Input: part model. Units: mm. Frame: model coordinates. A direction names the side the tool comes from. Give positions to 0.01 mm unless a question says otherwise; leave off trailing zeros. Order: outer loops, then holes, each group sorted by start corner. A loop starts at its lowest first (then second) coordinate and runs counter-clockwise, first axis right, second up. Notation, with made-up numbers: (-24, 9) - (25, 9) arc R19 cw to (25, 20) - close; hole circle Ø2 at (44, 14.25). An arc over 180 degrees is marked (long way). Answer in a Markdown table with one row per item. Add a question column.
1. Access query for faces 1 (the face through (-6.952, 0.493, -0.434)), 2 (the face through (1, 1, -1)). Directions: +Z, -Z, +X, -X, +Y, -Y. A direction counts if a zero-diameter tool reaches every point of the face in a straight line with its end or side. Return the directions, or none.
2. Ray query, line 1 (Y direction, x = -15.5, z = -58); line 2 (X direction, y = 65, z = 0); line 3 (Z direction, x = 53, y = 79). Return the intervals inside material, ascending. Write a range as [from, to].
3. Section query C-C on y = 13. Return loops of the section in (x, z), and give its area (3 significant figures).
4. Section query A-A on z = 0. Return loops of the section in (x, y), and give its area (3 significant figures).
5. Contact query for flat-ended pins moving along their axis: pin 1 (12 mm diameter, centred on y = 36.5, z = 1, fed in from +X); pin 2 (1.5 mm diameter, centred on x = -15.5, z = 31.5, fed in from +Y); pin 3 (3 mm diameter, centred on x = 34, y = 19, fed in from -Z). Output: stop coordinate, or through.
6. Section query B-B on x = 0. Return loops of the section in (y, z).
7. Mould query, pull axis X, two halves, no side actions, for faces 3 (the face through (-48, 100, 53.4)), 4 (the face through (-1.2, 0.5, -6.6)), 5 (the face through (21.477, 49.807, 68.198)), 6 (the face through (21.78, 49.3, 69.15)). Classes: released by +X, released by -X, zero draft, split by the parting line, or undercut.
8. Section query D-D on x = 22. Return loops of the section in (y, z), and give its area (3 significant figures).
```python
from build123d import *

# Parameters (mm, degrees)
SKETCH_6_R      = 71.5
SKETCH_6_R_2    = 2
EXTRUDE_2_DEPTH = 1
SKETCH_6_7_R    = 72.5
SKETCH_6_7_R_2  = 71.5
EXTRUDE_3_DEPTH = 100


with BuildPart() as part:
    # Sketch 6 → Extrude 2 (new body)
    with BuildSketch(Plane(origin=(0, 0, 0), x_dir=(1, 0, 0), z_dir=(0, 1, 0))):
        with Locations(Location((0, 0, 0), (0, 0, 270))):
            Circle(SKETCH_6_R)
        with Locations(Location((-5, 0, 0), (0, 0, 270))):
            Circle(SKETCH_6_R_2, mode=Mode.SUBTRACT)
        with Locations(Location((5, 0, 0), (0, 0, 270))):
            Circle(SKETCH_6_R_2, mode=Mode.SUBTRACT)
        with Locations(Location((0, 5, 0), (0, 0, 270))):
            Circle(SKETCH_6_R_2, mode=Mode.SUBTRACT)
        with Locations(Location((0, -5, 0), (0, 0, 270))):
            Circle(SKETCH_6_R_2, mode=Mode.SUBTRACT)
    extrude(amount=EXTRUDE_2_DEPTH)

    # Sketch 6_7 → Extrude 3 (add)
    with BuildSketch(Plane(origin=(0, 0, 0), x_dir=(1, 0, 0), z_dir=(0, 1, 0))):
        with Locations(Location((0, 0, 0), (0, 0, 270))):
            Circle(SKETCH_6_7_R)
        with Locations(Location((0, 0, 0), (0, 0, 270))):
            Circle(SKETCH_6_7_R_2, mode=Mode.SUBTRACT)
    extrude(amount=EXTRUDE_3_DEPTH)


solid = part.part
```
Answer:
| question | item | result |
|---|---|---|
| 1 | face 1 | +Y, -Y |
| 1 | face 2 | +Y |
| 2 | line 1 | y = [0, 1] |
| 2 | line 2 | x = [-72.5, -71.5], [71.5, 72.5] |
| 2 | line 3 | z = [-49.47, -47.99], [47.99, 49.47] |
| 3 | outline | circle Ø145 at (0, 0); hole circle Ø143 at (0, 0) |
| 3 | area | 452 mm² |
| 4 | outline | (-72.5, 0) - (-7, 0) - (-7, 1) - (-71.5, 1) - (-71.5, 100) - (-72.5, 100) - close; (-3, 0) - (3, 0) - (3, 1) - (-3, 1) - close; (7, 0) - (72.5, 0) - (72.5, 100) - (71.5, 100) - (71.5, 1) - (7, 1) - close |
| 4 | area | 335 mm² |
| 5 | pin 1 | stops at x = 72.5 |
| 5 | pin 2 | stops at y = 1 |
| 5 | pin 3 | stops at z = -64.81 |
| 6 | outline | (0, -72.5) - (100, -72.5) - (100, -71.5) - (1, -71.5) - (1, -7) - (0, -7) - close; (0, -3) - (1, -3) - (1, 3) - (0, 3) - close; (0, 7) - (1, 7) - (1, 71.5) - (100, 71.5) - (100, 72.5) - (0, 72.5) - close |
| 7 | face 3 | zero draft |
| 7 | face 4 | undercut |
| 7 | face 5 | undercut |
| 7 | face 6 | split by the parting line |
| 8 | outline | (0, -69.08) - (100, -69.08) - (100, -68.03) - (1, -68.03) - (1, 68.03) - (100, 68.03) - (100, 69.08) - (0, 69.08) - close |
| 8 | area | 346 mm² |
